Part model, mm, in its own coordinate system. Round coordinates to 2 decimals unless told otherwise and drop trailing zeros. Order: outer loops, then holes, each group sorted by start corner. A loop starts at its lowest first (then second) coordinate and runs counter-clockwise, first axis right, second up. Notation, with made-up numbers: (-18, 60.25) -> (29, 60.25) arc R19 ccw to (29, 87.25) -> close; hole circle Ø8 at (-3.5, 22). An arc over 180 degrees is marked (long way). Use CSV: the item, a comma, the result in double quotes.
```python
from build123d import *

# Parameters (mm, degrees)
F0_W     = 48
F0_H     = 69
F0_R     = 1.5
F1_DEPTH = 3
F2_W     = 34
F2_H     = 56
F3_DEPTH = 3
F4_R     = 5
F5_R     = 5


with BuildPart() as f1:
    # F0 (on Top) → F1 (new body)
    with BuildSketch(Plane.XY):
        Rectangle(F0_W, F0_H)
        with Locations((-21, -31.5)):
            Circle(F0_R, mode=Mode.SUBTRACT)
        with Locations((21, -31.5)):
            Circle(F0_R, mode=Mode.SUBTRACT)
        with Locations((-21, 31.5)):
            Circle(F0_R, mode=Mode.SUBTRACT)
        with Locations((21, 31.5)):
            Circle(F0_R, mode=Mode.SUBTRACT)
    extrude(amount=F1_DEPTH)

    # F2 (on face) → F3 (cut, through all)
    with BuildSketch(Plane.XY.offset(3)):
        Rectangle(F2_W, F2_H)
    extrude(amount=-F3_DEPTH, mode=Mode.SUBTRACT)

    # F4
    f4_edges = [f1.edges().sort_by_distance(p)[0] for p in [
        (-17, 28, 1.5),
    ]]
    fillet(f4_edges, radius=F4_R)

    # F5
    f5_edges = [f1.edges().sort_by_distance(p)[0] for p in [
        (-17, -28, 1.5),
        (17, -28, 1.5),
        (17, 28, 1.5),
    ]]
    fillet(f5_edges, radius=F5_R)


solid = f1.part
```
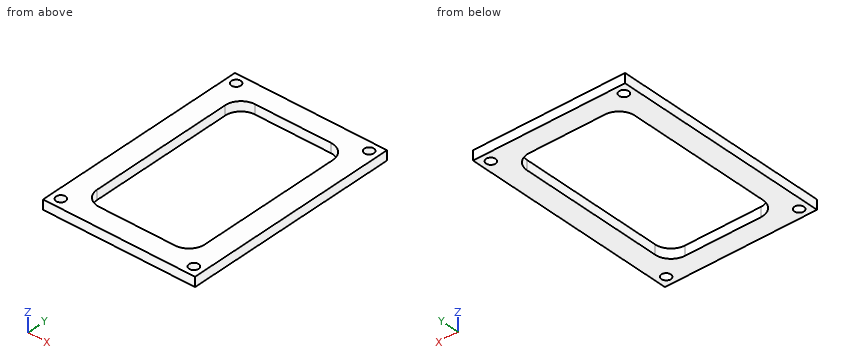
(1) Probe probe 1 along Y at (x, z) = (21, 2.45); probe 2 along Y at (x, z) = (1, 0.5); probe 3 along X at (y, z) = (14.5, 0.6). List the from-to ranges inside material, lowest first. Write a range as [from, to].
Reply:
probe 1,"[-34.5, -33], [-30, 30], [33, 34.5]"
probe 2,"[-34.5, -28], [28, 34.5]"
probe 3,"[-24, -17], [17, 24]"
(2) Drop flat-ended pins along their axis: P1, Ø5, axis at x = -21, y = 31.5, coming from the +Z side; P2, Ø1, axis at x = 15.5, y = -2.5, coming from the +Z side. Give the stop position or say it passes through.
Reply:
P1,"z = 3"
P2,"through"
(3) Cut at A-A, the plane x = -5. Give the cut face in (y, z).
Reply:
outline,"(-34.5, 0) -> (-28, 0) -> (-28, 3) -> (-34.5, 3) -> close; (28, 0) -> (34.5, 0) -> (34.5, 3) -> (28, 3) -> close"
(4) Cut at B-B, the plane y = 6.5. Give the cut face in (x, z), then the cut area to 3 significant figures.
Reply:
outline,"(-24, 0) -> (-17, 0) -> (-17, 3) -> (-24, 3) -> close; (17, 0) -> (24, 0) -> (24, 3) -> (17, 3) -> close"
area,"42.0 mm2"
(5) Cut at C-C, the plane z = 2.3. Give the cut face in (x, y), then the cut area to 3 significant figures.
Reply:
outline,"(-24, -34.5) -> (24, -34.5) -> (24, 34.5) -> (-24, 34.5) -> close; hole circle Ø3 at (-21, -31.5); hole circle Ø3 at (-21, 31.5); hole (-17, -23) arc R5 ccw to (-12, -28) -> (12, -28) arc R5 ccw to (17, -23) -> (17, 23) arc R5 ccw to (12, 28) -> (-12, 28) arc R5 ccw to (-17, 23) -> close; hole circle Ø3 at (21, -31.5); hole circle Ø3 at (21, 31.5)"
area,"1,400 mm2"
(6) Cut at D-D, the plane x = 21. Give the cut face in (y, z).
Reply:
outline,"(-34.5, 0) -> (-33, 0) -> (-33, 3) -> (-34.5, 3) -> close; (-30, 0) -> (30, 0) -> (30, 3) -> (-30, 3) -> close; (33, 0) -> (34.5, 0) -> (34.5, 3) -> (33, 3) -> close"
